Verification items for the finished model (mm, model axes). A direction names the side the tool comes from. Round coordinates to 2 decimals unless told otherwise and drop trailing zeros. Write each loop counter-clockwise with the first axis right and the second up, starting at its lowest first coordinate (ties: lowest second). Pieces come first, ordered by that corner, then holes. Notation, with made-up numbers: M 13.25,18 L 52.25,18 A25 ccw 52.25,32 Z; hole C 41,60.25 d8. An arc over 180 degrees is marked long. Use a Markdown table: item, result. Add a question column.
from build123d import *

# Parameters (mm, degrees)
SKETCH1_R           = 12
SKETCH1_R_2         = 1.5
BOSS_EXTRUDE1_DEPTH = 3.5
BOSS_EXTRUDE2_DEPTH = 8.3
SKETCH3_R           = 1.5
CUT_EXTRUDE1_DEPTH  = 19


with BuildPart() as part:
    # Sketch1 → Boss-Extrude1 (new body)
    with BuildSketch(Plane(origin=(0, 0, 0), x_dir=(1, 0, 0), z_dir=(0, 1, 0))):
        with Locations(Location((0, 0, 0), (0, 0, 270))):
            Circle(SKETCH1_R)
        with BuildLine():
            Line((2.598076211, 1.5), (2.598076211, -1.5))
            ThreePointArc((2.598076211, -1.5), (-2.974334584, -0.391578577), (2.121320344, 2.121320344))
            ThreePointArc((2.121320344, 2.121320344), (2.380060021, 1.826284287), (2.598076211, 1.5))
        make_face(mode=Mode.SUBTRACT)
        with Locations(Location((-6.363961031, -6.363961031, 0), (0, 0, 270))):
            Circle(SKETCH1_R_2, mode=Mode.SUBTRACT)
        with Locations(Location((6.363961031, -6.363961031, 0), (0, 0, 270))):
            Circle(SKETCH1_R_2, mode=Mode.SUBTRACT)
        with Locations(Location((-6.363961031, 6.363961031, 0), (0, 0, 270))):
            Circle(SKETCH1_R_2, mode=Mode.SUBTRACT)
        with Locations(Location((6.363961031, 6.363961031, 0), (0, 0, 270))):
            Circle(SKETCH1_R_2, mode=Mode.SUBTRACT)
    extrude(amount=BOSS_EXTRUDE1_DEPTH)

    # Sketch2 → Boss-Extrude2 (add)
    with BuildSketch(Plane(origin=(0, 3.5, 0), x_dir=(1, 0, 0), z_dir=(0, 1, 0))):
        with BuildLine():
            Line((4, -3), (4, 3))
            ThreePointArc((4, 3), (-5, 0), (4, -3))
        make_face()
        with BuildLine():
            Line((2.598076211, 1.5), (2.598076211, -1.5))
            ThreePointArc((2.598076211, -1.5), (-3, 0), (2.598076211, 1.5))
        make_face(mode=Mode.SUBTRACT)
    extrude(amount=BOSS_EXTRUDE2_DEPTH)

    # Sketch3 → Cut-Extrude1 (cut)
    with BuildSketch(Plane(origin=(4, 0, 0), x_dir=(0, 0, -1), z_dir=(1, 0, 0))):
        with Locations((0, 9.5)):
            Circle(SKETCH3_R)
    extrude(amount=-CUT_EXTRUDE1_DEPTH, mode=Mode.SUBTRACT)


solid = part.part
1. Scan lines: line 1 along Z through (x, y) = (0, 9.5); line 2 along Y through (x, z) = (-3.75, 0); line 3 along Y through (x, z) = (-9.75, -0.25). Record each from-to range of solid material in increasing order. Write a range as from..to.
2. Cross-section at B-B on x = 0. Enter the section's corners in (y, z).
3. Cross-section at A-A on z = 0. Enter the section's corners in (x, y), plus the area to 3 significant figures.
4. Depth check by flat-ended pin: pin 1 Ø1.8 at (y, z) = (6.5, 0.5) entering from +X; pin 2 Ø1.8 at (x, z) = (-6.36, -6.36) entering from +Y; pin 3 Ø3 at (x, y) = (-4.5, 4.5) entering from +Z; pin 4 Ø1 at (x, z) = (3, -7.5) entering from +Y. Enter the tip coordinate at first touch or a pass-through.
5. Release check for a two-part mould opening along Y. For faces 6 (the cylindrical face through (-6.94, 1.73, -4.98)), 7 (the cylindrical face through (3, 8, 0)), 8 (the flat face through (3, 0, 0)) record: +Y half, -Y half, draft (parallel to the pull), parting line (faces both ways), or undercut.
6. Access from +Z, -Z, +X, -X, +Y, -Y to the whole of each face (thin tool, end or side, straight path). Record for faces 1 (the flat face through (4, 7.6, 0)), 2 (the flat face through (2.598, 5, 0)), 3 (the cylindrical face through (-4, 8, 0)), 4 (the cylindrical face through (-4.997, 7.592, -0.175)), 5 (the flat face through (-3, 11.8, -2)).
7. Cross-section at C-C on x = 3. Enter the section's corners in (y, z).
8. Cross-section at D-D on y = 4.25. Enter the section's corners in (x, z).
Answer:
| question | item | result |
|---|---|---|
| 1 | line 1 | z = -5..-3, 3..5 |
| 1 | line 2 | y = 0..8, 11..11.8 |
| 1 | line 3 | y = 0..3.5 |
| 2 | outline | M 0,-12 L 3.5,-12 L 3.5,-5 L 11.8,-5 L 11.8,-3 L 0,-3 Z; M 0,3 L 11.8,3 L 11.8,5 L 3.5,5 L 3.5,12 L 0,12 Z |
| 3 | outline | M -12,0 L -3,0 L -3,8 L -5,8 L -5,3.5 L -12,3.5 Z; M -5,11 L -3,11 L -3,11.8 L -5,11.8 Z; M 2.6,0 L 12,0 L 12,3.5 L 4,3.5 L 4,8 L 2.6,8 Z; M 2.6,11 L 4,11 L 4,11.8 L 2.6,11.8 Z |
| 3 | area | 82.4 mm^2 |
| 4 | pin 1 | stops at x = 4 |
| 4 | pin 2 | passes through |
| 4 | pin 3 | stops at z = 11.51 |
| 4 | pin 4 | stops at y = 3.5 |
| 5 | face 6 | draft |
| 5 | face 7 | undercut |
| 5 | face 8 | -Y half |
| 6 | face 1 | +Z, -Z, +X, +Y |
| 6 | face 2 | +Y, -Y |
| 6 | face 3 | +X, -X |
| 6 | face 4 | +Y |
| 6 | face 5 | +Z, -Z, +X, -X, +Y |
| 7 | outline | M 0,-11.62 L 3.5,-11.62 L 3.5,-4 L 11.8,-4 L 11.8,4 L 3.5,4 L 3.5,11.62 L 0,11.62 Z; hole C 9.5,0 d3 |
| 8 | outline | M 4,-3 L 4,3 A5 ccw long Z; hole M 2.6,-1.5 L 2.6,1.5 A3 ccw long Z |
